Geometry check sheet. Reference: the model listing, model coordinates, mm. Face numbers are marked on the shaded views. Round coordinates to 2 decimals unless told otherwise and drop trailing zeros. Write each loop counter-clockwise with the first axis right and the second up, starting at its lowest first coordinate (ties: lowest second). Pieces come first, ordered by that corner, then holes. Notation, with made-up numbers: (32, 27) -> (90, 27) arc R26 ccw to (90, 65) -> close; hole circle Ø9 at (86, 41). An arc over 180 degrees is marked (long way). One line per question, with ' | ' between items.
Autodesk Inventor part; units mm, degrees
ref_plane "YZ Plane" through (0, 0, 0) normal (1, 0, 0) x (0, 1, 0)
ref_plane "XZ Plane" through (0, 0, 0) normal (0, 1, 0) x (-1, 0, 0)
ref_plane "XY Plane" through (0, 0, 0) normal (0, 0, 1) x (1, 0, 0)
sketch "Sketch1" plane through (0, 0, 0) normal (0, 1, 0) x (-1, 0, 0)
  circle A0 centre (0, 0) radius 12.7
  arc A1 (0, -15.875) -> (-15.875, 0) centre (0, 0) ccw
  line L0 (-15.875, -12.7) -> (-15.875, -16.51)
  line L1 (-15.875, -16.51) -> (0, -16.51)
  line L2 (0, -16.51) -> (0, -12.7)
  line L3 (-15.875, -12.7) -> (-15.875, 0)
  dimension "d0" = 25.4
  dimension "d1" = 31.75
  dimension "d2" = 3.81
extrude "Extrusion1" add sketch "Sketch1" along normal blind 25.4
sketch "Sketch2" plane through (15.875, 0, -16.51) normal (0, 0, -1) x (-1, 0, 0)
  circle A0 centre (7.9375, 12.7) radius 2.54
  line L0 (15.875, 0) -> (15.875, 25.4)
  dimension "d5" = 5.08
  dimension "d6" = 7.9375
extrude "Extrusion2" cut sketch "Sketch2" against normal blind 13.081
sketch "Sketch3" plane through (15.875, 0, -16.51) normal (0, 0, -1) x (-1, 0, 0)
  circle A0 centre (7.9375, 12.7) radius 3.175
  line L0 (15.875, 0) -> (15.875, 25.4)
  dimension "d9" = 6.35
  dimension "d10" = 7.9375
extrude "Extrusion3" cut sketch "Sketch3" against normal blind 5.08
properties part number "motor spinner"
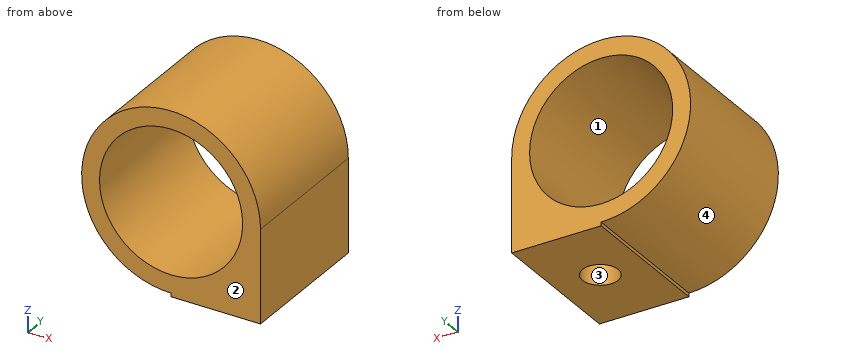
(1) Sectioned sample at B-B on z = 1. Record the cut outline in (x, y).
Resolved:
outline: (-15.84, 0) -> (-12.66, 0) -> (-12.66, 25.4) -> (-15.84, 25.4) -> close; (12.66, 0) -> (15.84, 0) -> (15.84, 25.4) -> (12.66, 25.4) -> close
(2) Sectioned sample at C-C on x = 12. Record the cut outline in (y, z), then the cut area to 3 significant figures.
Resolved:
outline: (0, -16.51) -> (25.4, -16.51) -> (25.4, -4.16) -> (0, -4.16) -> close; (0, 4.16) -> (25.4, 4.16) -> (25.4, 10.39) -> (0, 10.39) -> close | area: 472 mm2
(3) Material ranges on line 1 (X direction, y = 9.5, z = 0) (3 decimals); line 2 (Z direction, x = -9, y = 2.5); line 3 (X direction, y = 18, z = 3), recorded low to high.
Resolved:
line 1: x = -15.875 to -12.7, 12.7 to 15.875 | line 2: z = -13.08 to -8.96, 8.96 to 13.08 | line 3: x = -15.59 to -12.34, 12.34 to 15.59
(4) Draft check along X on the marked faces 1, 2, 3 and 4. Enter one of: +X half, -X half, draft (parallel to the pull), parting line (faces both ways), or undercut.
Resolved:
face 1: undercut | face 2: draft | face 3: undercut | face 4: parting line
(5) Sectioned sample at A-A on y = 23.25. Record the cut outline in (x, z) (3 decimals), then the cut area to 3 significant figures.
Resolved:
outline: (0, -16.51) -> (15.875, -16.51) -> (15.875, 0) arc R15.875 ccw (long way) to (0, -15.875) -> close; hole circle Ø25.4 at (0, 0) | area: 349 mm2
(6) Sectioned sample at D-D on x = 7. Record the cut outline in (y, z), then the cut area to 3 significant figures.
Resolved:
outline: (0, -16.51) -> (9.67, -16.51) -> (9.67, -11.43) -> (10.34, -11.43) -> (10.34, -10.6) -> (0, -10.6) -> close; (0, 10.6) -> (25.4, 10.6) -> (25.4, 14.25) -> (0, 14.25) -> close; (15.06, -11.43) -> (15.73, -11.43) -> (15.73, -16.51) -> (25.4, -16.51) -> (25.4, -10.6) -> (15.06, -10.6) -> close | area: 208 mm2
(7) Go/stop test with flat-tipped pins: pin 1 (5 mm diameter, centred on y = 13, z = 7.5, fed in from +X); pin 2 (5 mm diameter, centred on x = -5.5, y = 10.5, fed in from +Z); pin 3 (1.5 mm diameter, centred on y = 20, z = -5, fed in from -X). Record where each tip stops, or that it passes through.
Resolved:
pin 1: stops at x = 15.07 | pin 2: stops at z = 15.59 | pin 3: stops at x = -15.3
